Design review of the part shown in the three views and the two pictorial views. Dimensions are in mm from the part's minimum x, y and z. A direction names the side the tool comes from. Coordinates: 2 decimals unless noted, no trailing zeros. Loops run counter-clockwise (first coordinate to the right, second up) from the corner with the lowest first, then second, coordinate; pieces in that order, holes last. Notation, with made-up numbers: M -21.75,45.5 L 20.25,45.5 A23 ccw 20.25,82.5 Z; hole C 66.5,-12.5 d9. An arc over 180 degrees is marked long. Use one line per item in the form item = value.
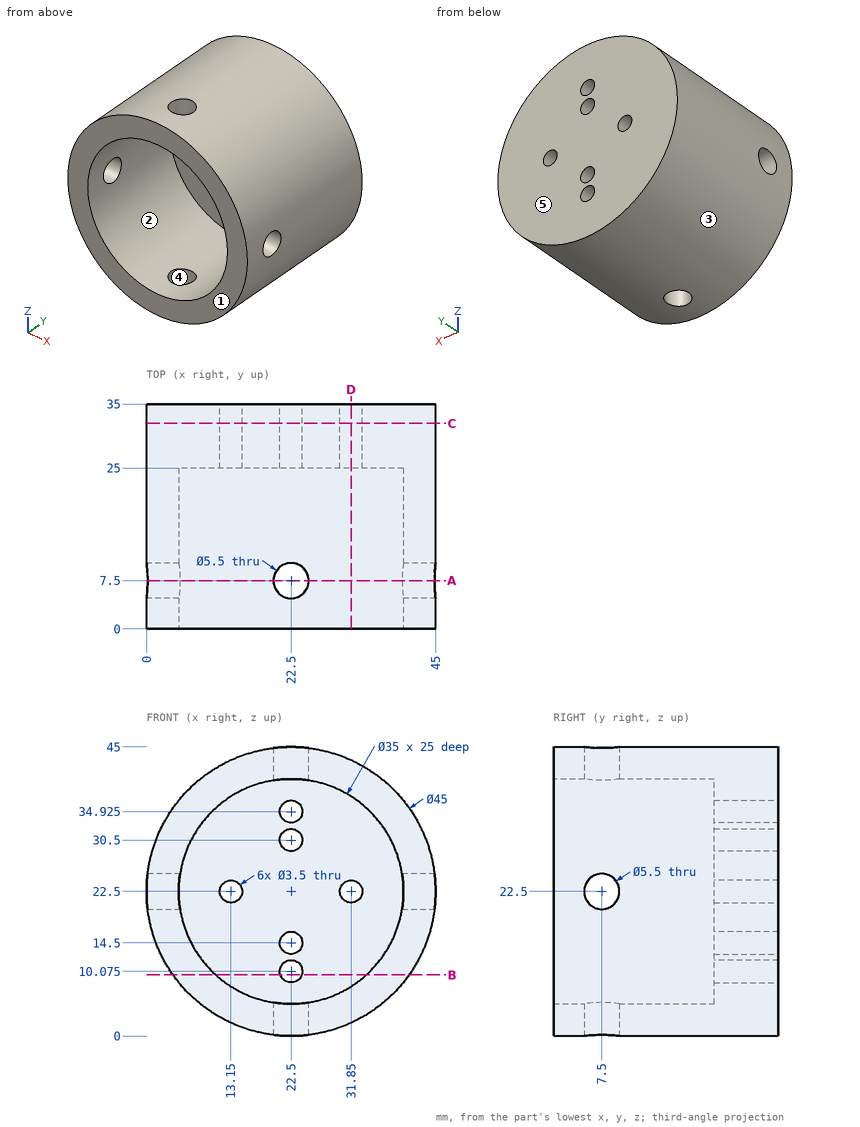
1. Machinability: for the marked faces 1 and 2, which of the approach directions +Z, -Z, +X, -X, +Y, -Y give a long, thin tool a straight path to every point of the face, cutting with its end or side? Answer none if there is none.
Response values:
face_1 = +Z, -Z, +X, -X, -Y
face_2 = -Y
2. Add section C-C (y = 32). State the section outline as (x, z) points (3 decimals), then the cut area to 3 significant figures.
Response values:
outline = C 22.5,22.5 d45; hole C 13.15,22.5 d3.5; hole C 22.5,10.075 d3.5; hole C 22.5,14.5 d3.5; hole C 22.5,30.5 d3.5; hole C 22.5,34.925 d3.5; hole C 31.85,22.5 d3.5
area = 1,530 mm^2
3. Insertion check: P1, Ø4.5, axis at x = 31.85, z = 22.5, coming from the -Y side; P2, Ø10, axis at y = 24, z = 12, coming from the +X side; P3, Ø12, axis at y = 17.5, z = 35.5, coming from the +X side. Each pin has a flat end and moves straight along its axis. Give the tip position at first contact, or say it passes through.
Response values:
P1 = 25
P2 = 44.32
P3 = 43.88
4. Wall thickness on line 1 along X through (y, z) = (7, 36); line 2 along Z through (x, y) = (17, 22.5); line 3 along X through (y, z) = (30, 31): over which ranges is each line inside the solid? List them lowest first. Write a range as from..to.
Response values:
line_1 = 4.5..11.36, 33.64..40.5
line_2 = 0.68..5.89, 39.11..44.32
line_3 = 1.67..20.82, 24.18..43.33
5. Add section D-D (x = 31.85). State the section outline as (y, z) points.
Response values:
outline = M 0,2.03 L 35,2.03 L 35,20.75 L 25,20.75 L 25,7.71 L 0,7.71 Z; M 0,37.29 L 25,37.29 L 25,24.25 L 35,24.25 L 35,42.97 L 0,42.97 Z
6. Add section B-B (z = 9.5). State the section outline as (x, y) points, then the cut area to 3 significant figures.
Response values:
outline = M 4.14,0 L 10.78,0 L 10.78,25 L 20.85,25 L 20.85,35 L 4.14,35 Z; M 24.15,25 L 34.22,25 L 34.22,0 L 40.86,0 L 40.86,35 L 24.15,35 Z
area = 667 mm^2
7. The part is to be moulded in two halves that separate along X. For the marked faces 3, 4 and 5, say which applies: pulls with the +X half, pulls with the -X half, needs draft (parallel to the pull), parting line crosses it, or undercut.
Response values:
face_3 = parting line crosses it
face_4 = undercut
face_5 = needs draft
8. Add section A-A (y = 7.5). State the section outline as (x, z) points.
Response values:
outline = M 0.17,19.75 A22.5 ccw 19.75,0.17 L 19.75,5.22 A17.5 cw 5.22,19.75 Z; M 0.17,25.25 L 5.22,25.25 A17.5 cw 19.75,39.78 L 19.75,44.83 A22.5 ccw Z; M 25.25,0.17 A22.5 ccw 44.83,19.75 L 39.78,19.75 A17.5 cw 25.25,5.22 Z; M 25.25,39.78 A17.5 cw 39.78,25.25 L 44.83,25.25 A22.5 ccw 25.25,44.83 Z
